from build123d import *

# Parameters (mm, degrees)
ESQUISSE1_R        = 1.5
BOSS_EXTRU_1_DEPTH = 3
CONG_2_R           = 2


with BuildPart() as part:
    # Esquisse1 → Boss.-Extru.1 (new body)
    with BuildSketch(Plane.XY):
        Polygon((-49.755710808, -4), (-9.749908145, 26.789473423), (6.665609221, -4), align=None)
        with Locations((-11.055921053, 20.736841844)):
            Circle(ESQUISSE1_R, mode=Mode.SUBTRACT)
        with Locations((-38, 0)):
            Circle(ESQUISSE1_R, mode=Mode.SUBTRACT)
        Circle(ESQUISSE1_R, mode=Mode.SUBTRACT)
    extrude(amount=BOSS_EXTRU_1_DEPTH)

    # Congé2
    cong_2_edges = [part.edges().sort_by_distance(p)[0] for p in [
        (-49.755710808, -4, 1.5),
        (-9.749908145, 26.789473423, 1.5),
        (6.665609221, -4, 1.5),
    ]]
    fillet(cong_2_edges, radius=CONG_2_R)


solid = part.part
Build history of the part. All positions in model axes, mm. Round coordinates to 2 decimals unless told otherwise and drop trailing zeros. Write each loop counter-clockwise with the first axis right and the second up, starting at its lowest first coordinate (ties: lowest second). Pieces come first, ordered by that corner, then holes. Notation, with made-up numbers: M 28,43.5 L 38,43.5 A8 ccw 38,54.5 Z; hole C -27.5,-9.5 d2. An arc over 180 degrees is marked long. Answer as a JSON object with one key per item and string values. Group by question number.
(1) Cut at C-C (x = 0). Give the cut face in (y, z), and give its area (3 significant figures).
(2) Drill centre lines: L1, parallel to X at y = 0.25, z = 1.4; L2, parallel to Y at x = 0, z = 1.15; L3, parallel to Y at x = -10, z = 1.8. Where is each one in solid material? Low to high.
(3) Cut at A-A (x = -38). Give the cut face in (y, z), and give its area (3 significant figures).
(4) Cut at D-D (y = 14.25). Give the cut face in (x, z).
(5) Mould opens along X. For faces 1 (the cylindrical face through (-10.005, 25.723, 1.521)), 2 (the cylindrical face through (-1.5, 0.07, 1.48)), 3 (the flat face through (-20, 8, 0)) say: pulls with the +X half, pulls with the -X half, needs draft (parallel to the pull), parting line crosses it, or undercut.
(6) Flat gauge pins, fed straight in: pin 1 (1.5 mm diameter, centred on y = 21, z = 2.5, fed in from +X); pin 2 (2.5 mm diameter, centred on x = -11.06, y = 20.74, fed in from +Z); pin 3 (1 mm diameter, centred on x = -20, z = 2, fed in from +Y). Where does each tip first touch, or does it go through?
(7) Cut at B-B (z = 2.05). Give the cut face in (x, y), and give its area (3 significant figures).
Responses:
{
 "1": {"outline": "M -4,0 L -1.5,0 L -1.5,3 L -4,3 Z; M 1.5,0 L 8.5,0 L 8.5,3 L 1.5,3 Z", "area": "28.5 mm2"},
 "2": {"L1": "x = -44.23 to -39.48, -36.52 to -1.48, 1.48 to 4.4", "L2": "y = -4 to -1.5, 1.5 to 8.5", "L3": "y = -4 to 19.67, 21.8 to 25.72"},
 "3": {"outline": "M -4,0 L -1.5,0 L -1.5,3 L -4,3 Z; M 1.5,0 L 5.05,0 L 5.05,3 L 1.5,3 Z", "area": "18.1 mm2"},
 "4": {"outline": "M -26.04,0 L -3.06,0 L -3.06,3 L -26.04,3 Z"},
 "5": {"face 1": "parting line crosses it", "face 2": "undercut", "face 3": "needs draft"},
 "6": {"pin 1": "stops at x = -6.26", "pin 2": "passes through", "pin 3": "stops at y = 19.29"},
 "7": {"outline": "M -45.1,-0.42 A2 ccw -43.88,-4 L 3.33,-4 A2 ccw 5.1,-1.06 L -8.64,24.7 A2 ccw -11.62,25.35 Z; hole C -38,0 d3; hole C -11.06,20.74 d3; hole C 0,0 d3", "area": "837 mm2"}
}
